CAD build for the part. Positions are in the model's coordinates, mm. A direction names the side the tool comes from. Give positions to 0.01 mm unless a question says otherwise; leave off trailing zeros. Order: outer loops, then holes, each group sorted by start corner. A loop starts at its lowest first (then second) coordinate and runs counter-clockwise, first axis right, second up.
```python
from build123d import *

# Parameters (mm, degrees)
F1_DEPTH = 26
F2_DEPTH = 20
F3_DEPTH = 4


with BuildPart() as f1:
    # F0 (on Front) → F1 (new body, symmetric)
    with BuildSketch(Plane.XZ):
        Polygon((-37.5, 0), (0, 0), (0, 9), (-5, 9), (-37.5, 9), align=None)
        Polygon((0, 9), (0, 0), (37.5, 0), (37.5, 9), (5, 9), align=None)
    extrude(amount=F1_DEPTH, both=True)

    # F0 (on Front) → F2 (join, symmetric)
    with BuildSketch(Plane.XZ):
        with BuildLine():
            Line((-5, 9), (0, 9))
            Line((0, 9), (0, 33.611993))
            Line((0, 33.611993), (0, 37))
            ThreePointArc((0, 37), (-8.485281, 40.514719), (-12, 49))
            Line((-12, 49), (-20, 49))
            ThreePointArc((-20, 49), (-15.811388, 36.752551), (-5, 29.635083))
            Line((-5, 29.635083), (-5, 9))
        make_face()
        with BuildLine():
            Line((0, 33.611993), (0, 9))
            Line((0, 9), (5, 9))
            Line((5, 9), (5, 29.635083))
            ThreePointArc((5, 29.635083), (15.811388, 36.752551), (20, 49))
            Line((20, 49), (12, 49))
            ThreePointArc((12, 49), (8.485281, 40.514719), (0, 37))
            Line((0, 37), (0, 33.611993))
        make_face()
    extrude(amount=F2_DEPTH, both=True)

    # F0 (on Front) → F3 (join, symmetric)
    with BuildSketch(Plane.XZ):
        with BuildLine():
            Line((-37.5, 9), (-5, 9))
            Line((-5, 9), (-5, 29.635083))
            ThreePointArc((-5, 29.635083), (-15.811388, 36.752551), (-20, 49))
            Line((-20, 49), (-37.5, 9))
        make_face()
        with BuildLine():
            Line((5, 9), (37.5, 9))
            Line((37.5, 9), (20, 49))
            ThreePointArc((20, 49), (15.811388, 36.752551), (5, 29.635083))
            Line((5, 29.635083), (5, 9))
        make_face()
    extrude(amount=F3_DEPTH, both=True)


solid = f1.part
```
Item 1: Slice it at B-B (y = 7). Give the cut face in (x, z).
Item 2: Tool access for faces 4 (the face through (17, 4, 25)), 5 (the face through (-18, -4, 20)), 6 (the face through (5, -12, 19)): list every direction of +Z, -Z, +X, -X, +Y, -Y with a clear straight run to the whole face (end or side of a thin tool).
Item 3: Two-plate mould, pull along Z, no slides. Class faces 1 (the face through (28.872, -0.056, 28.72)), 2 (the face through (0, -20, 29)), 3 (the face through (1, 22, 9)): released by +Z, released by -Z, zero draft, split by the parting line, or undercut.
Item 4: Slice it at A-A (z = 39). Give the cut face in (x, y) (1 decimal).
Item 5: Wall check: L1, parallel to Z at x = -16, y = -10; L2, parallel to Z at x = -9, y = 22; L3, parallel to X at y = -6, z = 16. Give the ranges that are in metal, low to high.
Item 6: Drop flat-ended pins along their axis: pin 1 Ø12 at (x, z) = (-10.5, 15.5) entering from +Y; pin 2 Ø8 at (y, z) = (9, 14.5) entering from -X; pin 3 Ø17.5 at (y, z) = (-15, 16) entering from +X; pin 4 Ø16 at (x, z) = (18.5, 19) entering from +Y. Give the stop position or say it passes through.
Item 7: Slice it at D-D (z = 34). Give the cut face in (x, y).
Item 8: Slice it at C-C (x = 18). Give the cut face in (y, z), and give its area (3 significant figures).
A:
1. outline: (-37.5, 0) - (37.5, 0) - (37.5, 9) - (5, 9) - (5, 29.64) arc R20 ccw to (20, 49) - (12, 49) arc R12 cw to (0, 37) arc R12 cw to (-12, 49) - (-20, 49) arc R20 ccw to (-5, 29.64) - (-5, 9) - (-37.5, 9) - close
2. face 4: +X, +Y
2. face 5: -X, -Y
2. face 6: +X, -Y
3. face 1: released by +Z
3. face 2: zero draft
3. face 3: undercut
4. outline: (-24.4, -4) - (-17.3, -4) - (-17.3, -20) - (-6.6, -20) - (-6.6, 20) - (-17.3, 20) - (-17.3, 4) - (-24.4, 4) - close; (6.6, -20) - (17.3, -20) - (17.3, -4) - (24.4, -4) - (24.4, 4) - (17.3, 4) - (17.3, 20) - (6.6, 20) - close
5. L1: z = 0 to 9, 37 to 49
5. L2: z = 0 to 9
5. L3: x = -5 to 5
6. pin 1: stops at y = 20
6. pin 2: stops at x = -5
6. pin 3: stops at x = 37.5
6. pin 4: stops at y = 4
7. outline: (-26.56, -4) - (-13.23, -4) - (-13.23, -20) - (13.23, -20) - (13.23, -4) - (26.56, -4) - (26.56, 4) - (13.23, 4) - (13.23, 20) - (-13.23, 20) - (-13.23, 4) - (-26.56, 4) - close
8. outline: (-26, 0) - (26, 0) - (26, 9) - (4, 9) - (4, 40.28) - (20, 40.28) - (20, 49) - (-20, 49) - (-20, 40.28) - (-4, 40.28) - (-4, 9) - (-26, 9) - close
8. area: 1,070 mm2
